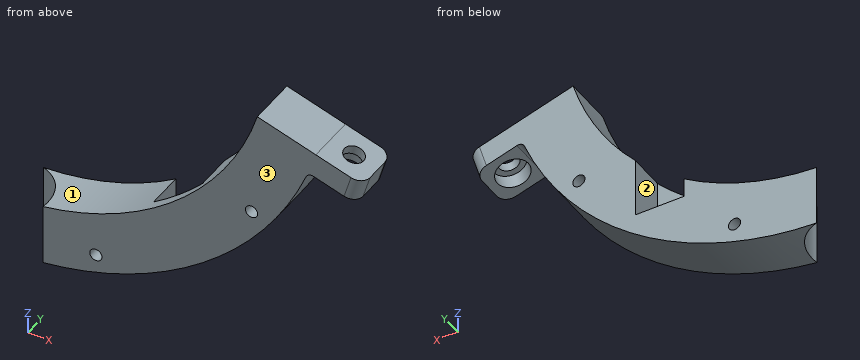
Autodesk Inventor part; units mm, degrees
ref_plane "YZ Plane" through (0, 0, 0) normal (1, 0, 0) x (0, 1, 0)
ref_plane "XZ Plane" through (0, 0, 0) normal (0, 1, 0) x (-1, 0, 0)
ref_plane "XY Plane" through (0, 0, 0) normal (0, 0, 1) x (1, 0, 0)
sketch "Sketch1" plane through (0, 0, 0) normal (0, 1, 0) x (-1, 0, 0)
  circle A0 centre (0, 0) radius 135
  circle A1 centre (0, 0) radius 110
  dimension "d0" = 270
  dimension "d1" = 220
extrude "Extrusion1" add sketch "Sketch1" along normal mid plane 47
sketch "Sketch2" plane through (0, 0, 0) normal (0, 0, 1) x (1, 0, 0)
  circle A0 centre (0, -20.5) radius 18
  line L0 (-135, -23.5) -> (135, -23.5)
  dimension "d4" = 36
  dimension "d38" = 3
extrude "Extrusion2" cut sketch "Sketch2" against normal through all
sketch "Sketch3" plane through (0, 23.5, 0) normal (0, 1, 0) x (1, 0, 0)
  circle A0 centre (0, 0) radius 127.5
  circle A1 centre (-127.5, 0) radius 2
  circle A2 centre (-103.1497, -74.9426) radius 2
  circle A3 centre (-39.3997, -121.2597) radius 2
  circle A4 centre (39.3997, -121.2597) radius 2
  circle A5 centre (103.1497, -74.9426) radius 2
  circle A6 centre (127.5, 0) radius 2
  circle A7 centre (103.1497, 74.9426) radius 2
  circle A8 centre (39.3997, 121.2597) radius 2
  circle A9 centre (-39.3997, 121.2597) radius 2
  circle A10 centre (-103.1497, 74.9426) radius 2
  dimension "d7" = 255
  dimension "d8" = 4
  dimension "d11" = 360
hole "Hole1" at (39.3997, 23.5, 121.2597) at (-39.3997, 23.5, 121.2597) at (-103.1497, 23.5, 74.9426) at (-127.5, 23.5, 0) at (-103.1497, 23.5, -74.9426) at (-39.3997, 23.5, -121.2597) at (39.3997, 23.5, -121.2597) at (103.1497, 23.5, -74.9426) at (127.5, 23.5, 0) at (103.1497, 23.5, 74.9426) direction (0, -1, 0) diameter 5 end through all
sketch "Sketch4" plane through (0, 23.5, 0) normal (0, 1, 0) x (1, 0, 0)
  circle A0 centre (0, 0) radius 140
extrude "Extrusion3" cut sketch "Sketch4" against normal blind 27
sketch "Sketch7" plane through (0, -3.5, 0) normal (0, 1, 0) x (1, 0, 0)
  line L0 (0, 0) -> (70, 0)
  line L1 (80, -100) -> (60, -100)
  line L2 (60, -100) -> (60, 100)
  line L3 (60, 100) -> (80, 100)
  line L4 (80, 100) -> (80, -100)
  line L5 (80, -100) -> (60, 100) construction
  line L6 (60, -100) -> (80, 100) construction
  dimension "d39" = 70
  dimension "d40" = 20
  dimension "d41" = 200
extrude "Extrusion7" cut sketch "Sketch7" against normal blind 15
sketch "Sketch8" plane through (0, -3.5, 0) normal (0, 1, 0) x (1, 0, 0)
  line L0 (-129.4827, -38.1999) -> (129.4827, 38.1999)
  line L1 (0, 134.8703) -> (0, -135)
  arc A0 (-5.9161, 134.8703) -> (5.9161, 134.8703) centre (0, 0) ccw
extrude "Extrusion8" cut sketch "Sketch8" against normal through all
sketch "Sketch9" plane through (0, -3.5, 0) normal (0, 1, 0) x (1, 0, 0)
  line L0 (-129.4827, -38.1999) -> (-105.5044, -31.1258)
  arc A0 (-5.9161, 109.8408) -> (-105.5044, -31.1258) centre (0, 0) ccw
  line L1 (-5.9161, 134.8703) -> (-5.9161, 109.8408)
  arc A1 (-5.9161, 134.8703) -> (-129.4827, -38.1999) centre (0, 0) ccw
  circle A2 centre (-39.3997, 121.2597) radius 2.5
  circle A3 centre (-103.1497, 74.9426) radius 2.5
  circle A4 centre (-127.5, 0) radius 2.5
extrude "Extrusion9" cut sketch "Sketch9" against normal through all
sketch "Sketch10" plane through (129.4827, -23.5, -38.1999) normal (0.2829619, 0, 0.9591312) x (0.9591312, 0, -0.2829619)
  line L0 (0, 0) -> (-25, 0)
  line L1 (-2.5, 0) -> (15, 0)
  line L2 (20, 5) -> (20, 15)
  line L3 (15, 20) -> (-2.5, 20)
  line L4 (-2.5, 20) -> (-2.5, 0)
  line L5 (0, 20) -> (0, 0)
  arc A0 (20, 15) -> (15, 20) centre (15, 15) ccw
  arc A1 (15, 0) -> (20, 5) centre (15, 5) ccw
  point P0 (-135, 23.5)
  point P1 (20, 20)
  point P2 (20, 0)
  point P3 (0, 0)
  dimension "d48" = 22.5
  dimension "d49" = 20
  dimension "d50" = 20
  dimension "d53" = 5
extrude "Extrusion10" add sketch "Sketch10" against normal blind 10
fillet "Fillet1" radius 2.5 1 edges at (126.2974, -13.5, -47.6862)
sketch "Sketch11" plane through (126.6531, -23.5, -47.7912) normal (-0.2829619, 0, -0.9591312) x (-0.9591312, 0, 0.2829619)
  line L0 (-1.9306, 20) -> (-15, 20)
  line L1 (-20, 15) -> (-20, 5)
  point P0 (135, 23.5)
  point P1 (-10, 10)
  dimension "d55" = 10
  dimension "d56" = 10
hole "Hole2" at (136.2444, -13.5, -50.6208) direction (0.2829619, 0, 0.9591312) diameter 8.2 end through all counterbore diameter 13.2 counterbore depth 6
properties part number "Cylinder Spacer Bottom_Q2"
Can you work these out from the model? Positions are in its coordinate system, mm. Face numbers are marked on the shaded views. Coordinates: 2 decimals unless noted, no trailing zeros. Loops run counter-clockwise (first coordinate to the right, second up) from the corner with the lowest first, then second, coordinate; pieces in that order, holes last. Notation, with made-up numbers: (24.25, 81.5) -> (82.25, 81.5) arc R29 ccw to (82.25, 112.5) -> close; hole circle Ø9 at (0.25, 58.25). An arc over 180 degrees is marked (long way). Answer as a JSON object with one key per item and string values.
1) Imagine slicing it at B-B (x = 62). Please give me the cut outline in (y, z), then the cut area to 3 significant figures.
Results:
{"outline": "(-23.5, -119.92) -> (-3.5, -119.92) -> (-3.5, -100) -> (-18.5, -100) -> (-18.5, -90.86) -> (-23.5, -90.86) -> close", "area": "444 mm^2"}
2) Thinking about a two-plate mould opening in X: for the marked faces 1, 2 and 3, which applies, pulls with the +X half, pulls with the -X half, needs draft (parallel to the pull), parting line crosses it, or undercut?
Results:
{"face 1": "pulls with the -X half", "face 2": "undercut", "face 3": "needs draft"}
3) Imagine slicing it at C-C (z = -98). Please give me the cut outline in (x, y).
Results:
{"outline": "(49.96, -23.5) -> (92.85, -23.5) -> (92.85, -3.5) -> (80, -3.5) -> (80, -18.5) -> (60, -18.5) -> (60, -3.5) -> (49.96, -3.5) -> close"}
4) Imagine slicing it at A-A (z = -121). Please give me the cut outline in (x, y).
Results:
{"outline": "(5.92, -3.5) arc R18 cw to (17.75, -23.5) -> (36.91, -23.5) -> (36.91, -3.5) -> close; (41.89, -23.5) -> (59.87, -23.5) -> (59.87, -3.5) -> (41.89, -3.5) -> close"}
5) If I drill on line 1 (X direction, y = -18, z = -119.5); line 2 (Z direction, x = 40.5, y = -7.5); line 3 (X direction, y = -16.5, z = -96.5), over which ranges is the centre line in solid material (lowest first)?
Results:
{"line 1": "x = 17.83 to 37.62, 41.18 to 62.81", "line 2": "z = -128.78 to -123.5, -119.01 to -102.27", "line 3": "x = 52.8 to 60, 80 to 94.41"}
6) For P1, Ø8, axis at x = 36, y = -16.5, coming from the -Z side; P2, Ø5, axis at x = 51, y = -8, coming from the -Z side; P3, Ø5, axis at x = 106.5, y = -14.5, coming from the -Z side, each with a flat end and sliding along its axis, tell me the tip position at first contact or that it passes through.
Results:
{"P1": "stops at z = -131.15", "P2": "stops at z = -125.99", "P3": "stops at z = -86.08"}
7) Imagine slicing it at D-D (x = 26). Please give me the cut outline in (y, z), then the cut area to 3 significant figures.
Results:
{"outline": "(-23.5, -132.47) -> (-3.5, -132.47) -> (-3.5, -106.88) -> (-23.5, -106.88) -> close", "area": "512 mm^2"}
